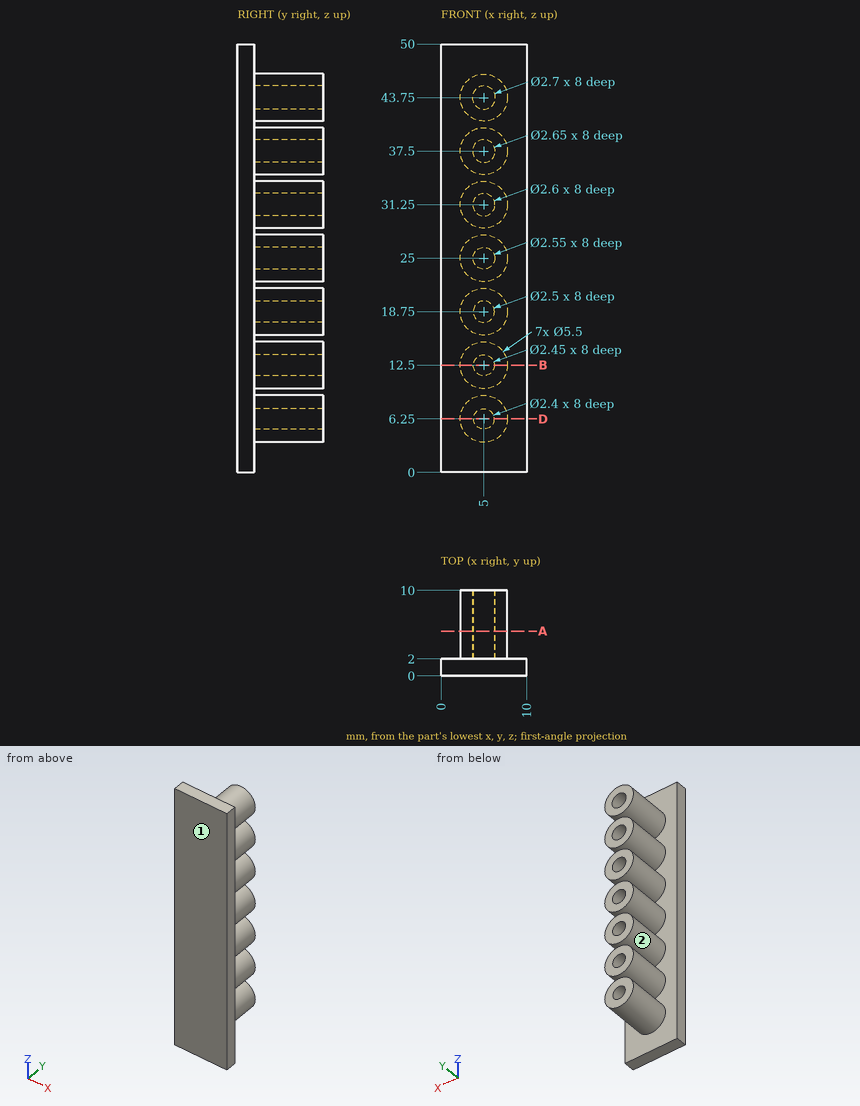
The figure shows three views and two pictorial views of one solid part (mm, origin at its lowest corner). Answer the questions. A direction names the side the tool comes from. Round coordinates to 2 decimals unless told otherwise and drop trailing zeros. Write each loop counter-clockwise with the first axis right and the second up, starting at its lowest first coordinate (ties: lowest second). Pieces come first, ordered by that corner, then holes. Notation, with made-up numbers: M -31,-7 L -19,-7 A19 cw -19,21 Z; hole C -32,19.5 d8. An arc over 180 degrees is marked long. Use a Markdown table: item, result.
1) The part is cut by section D-D on z = 6.25. Give the vertices of the cut face in (x, y).
Taken from the geometry:
| item | result |
|---|---|
| outline | M 0,0 L 10,0 L 10,2 L 7.75,2 L 7.75,10 L 6.2,10 L 6.2,2 L 3.8,2 L 3.8,10 L 2.25,10 L 2.25,2 L 0,2 Z |
2) The part is cut by section A-A on y = 5.25. State how many separate pieces and enclosed holes the cut face has, plus the area to 3 significant figures.
Taken from the geometry:
| item | result |
|---|---|
| separate pieces | 7 |
| enclosed holes | 7 |
| area | 131 mm2 |
3) Flat-ended cylindrical pins translate along their axes: pin 1 (1.3 mm diameter, centred on x = 5.5, z = 37.5, fed in from +Y); pin 2 (3 mm diameter, centred on x = 5.5, z = 31.5, fed in from +Y); pin 3 (3 mm diameter, centred on x = 5.5, y = 4, fed in from +Z); pin 4 (1.5 mm diameter, centred on y = 7.5, z = 36.5, fed in from -X). Find the tip coordinate at first contact, or state that the pin passes through.
Taken from the geometry:
| item | result |
|---|---|
| pin 1 | stops at y = 2 |
| pin 2 | stops at y = 10 |
| pin 3 | stops at z = 46.5 |
| pin 4 | stops at x = 2.26 |
4) The part is cut by section B-B on z = 12.5. Give the vertices of the cut face in (x, y) (3 decimals).
Taken from the geometry:
| item | result |
|---|---|
| outline | M 0,0 L 10,0 L 10,2 L 7.75,2 L 7.75,10 L 6.225,10 L 6.225,2 L 3.775,2 L 3.775,10 L 2.25,10 L 2.25,2 L 0,2 Z |
5) Which of the six approach directions +Z, -Z, +X, -X, +Y, -Y give full straight-line access (tool end or side, diameter ignored) to the marked faces 1 and 2?
Taken from the geometry:
| item | result |
|---|---|
| face 1 | +Z, -Z, +X, -X, -Y |
| face 2 | +Y |
6) Consider line 1 (X direction, y = 5, z = 43.75); line 2 (Y direction, x = 7.5, z = 10.5); line 3 (X direction, y = 7, z = 23.5). Determine where each line is inside the solid, lowest interval first. Write a range as [from, to].
Taken from the geometry:
| item | result |
|---|---|
| line 1 | x = [2.25, 3.65], [6.35, 7.75] |
| line 2 | y = [0, 2] |
| line 3 | x = [2.7, 7.3] |
